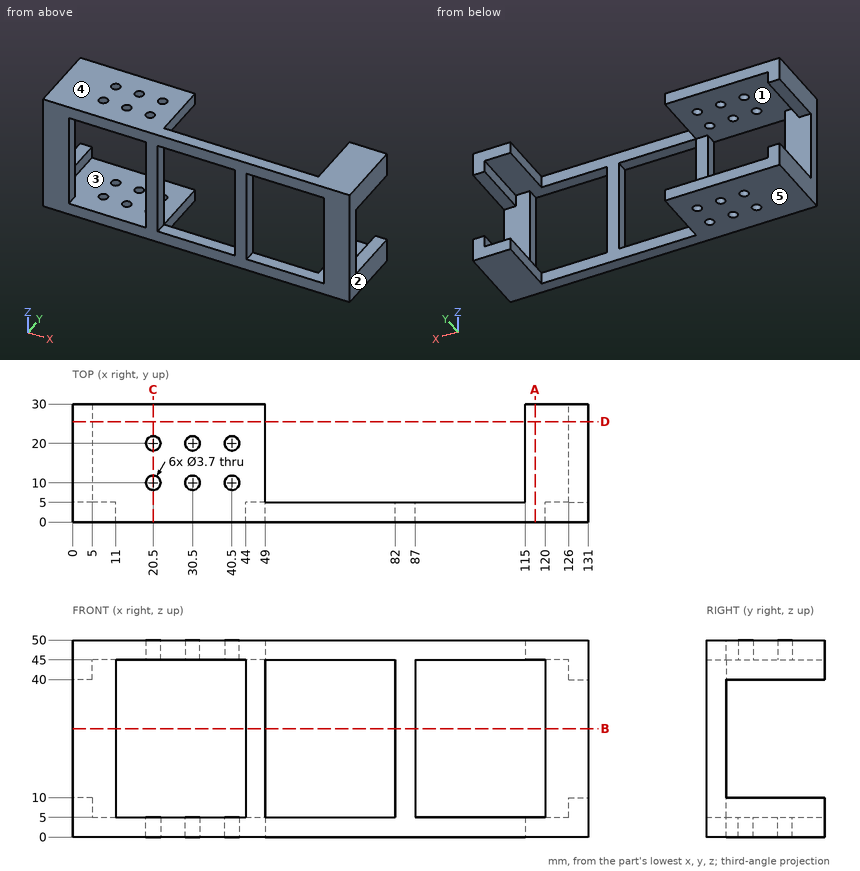
Job drawing, mm, ordinate dimensions from the low corner. One solid piece. A direction names the side the tool comes from. Coordinates: 2 decimals unless noted, no trailing zeros. Loops run counter-clockwise (first coordinate to the right, second up) from the corner with the lowest first, then second, coordinate; pieces in that order, holes last. Notation, with made-up numbers: (82, 42.25) -> (113, 42.25) arc R34 ccw to (113, 73.25) -> close; hole circle Ø4 at (70, 57.25). An arc over 180 degrees is marked (long way). One line per item, written item: value.
1. Which spindle directions (+Z, -Z, +X, -X, +Y, -Y) get a long thin tool onto all of the face, cutting with end or side? Do the marked faces 1 and 2. Say none if no direction does.
Answers:
face 1: +Y
face 2: +Z, -Z, +X, +Y, -Y
2. Slice it at C-C on x = 20.5. Write the cut outline in (y, z), and give its area (3 significant figures).
Answers:
outline: (0, 0) -> (8.15, 0) -> (8.15, 5) -> (0, 5) -> close; (0, 45) -> (8.15, 45) -> (8.15, 50) -> (0, 50) -> close; (11.85, 0) -> (18.15, 0) -> (18.15, 5) -> (11.85, 5) -> close; (11.85, 45) -> (18.15, 45) -> (18.15, 50) -> (11.85, 50) -> close; (21.85, 0) -> (30, 0) -> (30, 5) -> (21.85, 5) -> close; (21.85, 45) -> (30, 45) -> (30, 50) -> (21.85, 50) -> close
area: 226 mm^2
3. Pull direction Z, two halves, no side cores. Call the marked faces 3, 4 and 5: pulls with the +Z half, pulls with the -Z half, needs draft (parallel to the pull), parting line crosses it, or undercut.
Answers:
face 3: undercut
face 4: pulls with the +Z half
face 5: pulls with the -Z half
4. Slice it at D-D on y = 25.5. Write the cut outline in (x, z).
Answers:
outline: (0, 0) -> (49, 0) -> (49, 5) -> (5, 5) -> (5, 10) -> (0, 10) -> close; (0, 40) -> (5, 40) -> (5, 45) -> (49, 45) -> (49, 50) -> (0, 50) -> close; (115, 0) -> (131, 0) -> (131, 10) -> (126, 10) -> (126, 5) -> (115, 5) -> close; (115, 45) -> (126, 45) -> (126, 40) -> (131, 40) -> (131, 50) -> (115, 50) -> close
5. Slice it at B-B on z = 27.5. Write the cut outline in (x, y), and give its area (3 significant figures).
Answers:
outline: (0, 0) -> (11, 0) -> (11, 5) -> (0, 5) -> close; (44, 0) -> (49, 0) -> (49, 5) -> (44, 5) -> close; (82, 0) -> (87, 0) -> (87, 5) -> (82, 5) -> close; (120, 0) -> (131, 0) -> (131, 5) -> (120, 5) -> close
area: 160 mm^2
6. Slice it at A-A on x = 117.5. Write the cut outline in (y, z).
Answers:
outline: (0, 0) -> (30, 0) -> (30, 5) -> (0, 5) -> close; (0, 45) -> (30, 45) -> (30, 50) -> (0, 50) -> close
7. Drill centre lines: line 1 (X direction, y = 20, z = 48.6); line 2 (Y direction, x = 20.5, z = 1.05); line 3 (X direction, y = 22.5, z = 41). Where is each one in solid material? Low to high. Write a range as [from, to].
Answers:
line 1: x = [0, 18.65], [22.35, 28.65], [32.35, 38.65], [42.35, 49], [115, 131]
line 2: y = [0, 8.15], [11.85, 18.15], [21.85, 30]
line 3: x = [0, 5], [126, 131]
8. Flat gauge pins, fed straight in: P1, Ø3.5, axis at x = 20.5, y = 10, coming from the -Z side; P2, Ø12, axis at x = 4, z = 32, coming from the +Y side. Where does each tip first touch, or does it go through?
Answers:
P1: passes through
P2: stops at y = 5
